from build123d import *

# Parameters (mm, degrees)
BOSS_EXTRUDE1_DEPTH = 6
SKETCH2_R           = 2.6
BOSS_EXTRUDE2_DEPTH = 1.5
CHAMFER1_SIZE       = 2
CHAMFER2_SIZE       = 6


with BuildPart() as part:
    # Sketch1 → Boss-Extrude1 (new body)
    with BuildSketch(Plane(origin=(0, 0, 789.620141885), x_dir=(-1, 0, 0), z_dir=(0, 0, -1))):
        with BuildLine():
            Line((8.210843614, -513.298939869), (8.210843614, -527.298939869))
            Line((8.210843614, -527.298939869), (10.210843614, -529.298939869))
            Line((10.210843614, -529.298939869), (25.210843614, -529.298939869))
            Line((25.210843614, -529.298939869), (25.210843614, -520.298939869))
            ThreePointArc((25.210843614, -520.298939869), (31.210843614, -514.298939869), (37.210843614, -520.298939869))
            Line((37.210843614, -520.298939869), (37.210843614, -529.298939869))
            Line((37.210843614, -529.298939869), (52.210843614, -529.298939869))
            Line((52.210843614, -529.298939869), (54.210843614, -527.298939869))
            Line((54.210843614, -527.298939869), (54.210843614, -513.298939869))
            Line((54.210843614, -513.298939869), (52.210843614, -511.298939869))
            Line((52.210843614, -511.298939869), (10.210843614, -511.298939869))
            Line((10.210843614, -511.298939869), (8.210843614, -513.298939869))
        make_face()
        Polygon((10.960843614, -517.845201225), (10.960843614, -522.752678513), (15.210843614, -525.206417157), (19.460843614, -522.752678513), (19.460843614, -517.845201225), (15.210843614, -515.391462581), align=None, mode=Mode.SUBTRACT)
        Polygon((47.210843614, -515.391462581), (42.960843614, -517.845201225), (42.960843614, -522.752678513), (47.210843614, -525.206417157), (51.460843614, -522.752678513), (51.460843614, -517.845201225), align=None, mode=Mode.SUBTRACT)
    extrude(amount=BOSS_EXTRUDE1_DEPTH)

    # Sketch2 → Boss-Extrude2 (add)
    # profile 1 of 2: a face of its own
    with BuildSketch(Plane.XY.offset(789.620141885)):
        Polygon((-10.960843614, -517.845201225), (-15.210843614, -515.391462581), (-19.460843614, -517.845201225), (-19.460843614, -522.752678513), (-15.210843614, -525.206417157), (-10.960843614, -522.752678513), align=None)
        with Locations((-15.210843614, -520.298939869)):
            Circle(SKETCH2_R, mode=Mode.SUBTRACT)
    # profile 2 of 2: a face of its own
    with BuildSketch(Plane.XY.offset(789.620141885)):
        Polygon((-47.210843614, -515.391462581), (-51.460843614, -517.845201225), (-51.460843614, -522.752678513), (-47.210843614, -525.206417157), (-42.960843614, -522.752678513), (-42.960843614, -517.845201225), align=None)
        with Locations((-47.210843614, -520.298939869)):
            Circle(SKETCH2_R, mode=Mode.SUBTRACT)
    extrude(amount=-BOSS_EXTRUDE2_DEPTH)

    # Chamfer1
    chamfer1_edges = [part.edges().sort_by_distance(p)[0] for p in [
        (-25.210843614, -529.298939869, 786.620141885),
        (-37.210843614, -529.298939869, 786.620141885),
    ]]
    chamfer(chamfer1_edges, length=CHAMFER1_SIZE)

    # Chamfer2
    # the kernel refuses this chamfer: 6 mm, written as the material it takes off along each edge
    with BuildSketch(Plane(origin=(-67.640941541, -511.298939869, 783.620141885), x_dir=(0, 0.027495876610582292, 0.9996219169112969), z_dir=(1, 0, 0))) as chamfer2_piece_1:
        Polygon((CHAMFER2_SIZE * 0.999621916911, CHAMFER2_SIZE * 0.0274958766106), (-CHAMFER2_SIZE * 0.0274958766106, CHAMFER2_SIZE * 0.999621916911), (0, 0), align=None)
    extrude(amount=72.860195856, mode=Mode.SUBTRACT)


solid = part.part
Work out the finished part from the listing and answer in its coordinate system (mm). A direction names the side the tool comes from. Round coordinates to 2 decimals unless told otherwise and drop trailing zeros. Write each loop counter-clockwise with the first axis right and the second up, starting at its lowest first coordinate (ties: lowest second). Pieces come first, ordered by that corner, then holes.
1) Given pin 1 Ø6 at (x, y) = (-47.21, -520.3) entering from -Z; pin 2 Ø1 at (x, z) = (-28, 786) entering from -Y; pin 3 Ø3 at (x, y) = (-15.21, -520.3) entering from +Z, each flat-ended and moving along its own axis, determine where each tip first touches the part or whether it passes through.
2) A cutting plane is placed at C-C (z = 784.5). Give the vertices of the cut face in (x, y), plus the area to 3 significant figures.
3) Straight lines are drawn through the part: line 1 (X direction, y = -522.25, z = 785.5); line 2 (X direction, y = -526.25, z = 786.5); line 3 (X direction, y = -518, z = 789). For each, find the intervals that lie inside material, in ascending order.
4) The mould has two halves that part along Y. Classify faces 4 (the flat face through (-54.211, -520, 787)), 5 (the flat face through (-13.12, -516.6, 786.4)), 6 (the flat face through (-53.45, -512.54, 788.86)): pulls with the +Y half, pulls with the -Y half, needs draft (parallel to the pull), parting line crosses it, or undercut.
5) A cutting plane is placed at A-A (y = -516.5). Give the vertices of the cut face in (x, z).
6) A tool of negligible diameter and unlimited length cuts with its end or side. For faces 1 (the flat face through (-25.211, -524, 787)), 2 (the cylindrical face through (-47.55, -517.72, 788.88)), 3 (the flat face through (-45.12, -516.6, 786.4)), from which of +Z, -Z, +X, -X, +Y, -Y can it reach the whole face along a straight path? Write none if from no direction.
7) A cutting plane is placed at B-B (z = 788.75). Give the vertices of the cut face in (x, y).
8) A cutting plane is placed at D-D (y = -522.25). Give the vertices of the cut face in (x, z), plus the area to 3 significant figures.
Completed:
1. pin 1: stops at z = 788.12
1. pin 2: stops at y = -515.58
1. pin 3: passes through
2. outline: (-54.21, -527.3) - (-52.21, -529.3) - (-39.21, -529.3) - (-37.21, -527.3) - (-37.21, -520.3) arc R6 cw to (-35.79, -516.42) - (-45.43, -516.42) - (-42.96, -517.85) - (-42.96, -522.75) - (-47.21, -525.21) - (-51.46, -522.75) - (-51.46, -517.85) - (-48.99, -516.42) - (-54.21, -516.42) - close; (-26.63, -516.42) arc R6 cw to (-25.21, -520.3) - (-25.21, -527.3) - (-23.21, -529.3) - (-10.21, -529.3) - (-8.21, -527.3) - (-8.21, -516.42) - (-13.43, -516.42) - (-10.96, -517.85) - (-10.96, -522.75) - (-15.21, -525.21) - (-19.46, -522.75) - (-19.46, -517.85) - (-16.99, -516.42) - close
2. area: 312 mm2
3. line 1: x = -54.21 to -51.46, -42.96 to -37.21, -25.21 to -19.46, -10.96 to -8.21
3. line 2: x = -54.21 to -37.21, -25.21 to -8.21
3. line 3: x = -54.21 to -48.43, -46 to -36.75, -25.67 to -16.43, -14 to -8.21
4. face 4: needs draft
4. face 5: undercut
4. face 6: pulls with the +Y half
5. outline: (-54.21, 784.42) - (-49.13, 784.42) - (-49.13, 788.12) - (-45.29, 788.12) - (-45.29, 784.42) - (-35.85, 784.42) - (-35.85, 789.62) - (-54.21, 789.62) - close; (-26.57, 784.42) - (-17.13, 784.42) - (-17.13, 788.12) - (-13.29, 788.12) - (-13.29, 784.42) - (-8.21, 784.42) - (-8.21, 789.62) - (-26.57, 789.62) - close
6. face 1: +Z, -Z, -Y
6. face 2: +Z, -Z
6. face 3: -Z
7. outline: (-54.21, -527.3) - (-52.21, -529.3) - (-39.21, -529.3) - (-37.21, -527.3) - (-37.21, -520.3) arc R6 cw to (-25.21, -520.3) - (-25.21, -527.3) - (-23.21, -529.3) - (-10.21, -529.3) - (-8.21, -527.3) - (-8.21, -513.3) - (-9.34, -512.17) - (-53.08, -512.17) - (-54.21, -513.3) - close; hole circle Ø5.2 at (-47.21, -520.3); hole circle Ø5.2 at (-15.21, -520.3)
8. outline: (-54.21, 783.62) - (-51.46, 783.62) - (-51.46, 788.12) - (-48.93, 788.12) - (-48.93, 789.62) - (-54.21, 789.62) - close; (-45.49, 788.12) - (-42.96, 788.12) - (-42.96, 783.62) - (-37.21, 783.62) - (-37.21, 789.62) - (-45.49, 789.62) - close; (-25.21, 783.62) - (-19.46, 783.62) - (-19.46, 788.12) - (-16.93, 788.12) - (-16.93, 789.62) - (-25.21, 789.62) - close; (-13.49, 788.12) - (-10.96, 788.12) - (-10.96, 783.62) - (-8.21, 783.62) - (-8.21, 789.62) - (-13.49, 789.62) - close
8. area: 117 mm2
